Geometry: final body of the model. Coordinates: model frame, mm. Face numbers are marked on the shaded views. A direction names the side the tool comes from. Give positions to 0.01 mm unless a question says otherwise; leave off trailing zeros. Write each loop counter-clockwise with the first axis right and the second up, starting at its lowest first coordinate (ties: lowest second). Pieces come first, ordered by that corner, then holes.
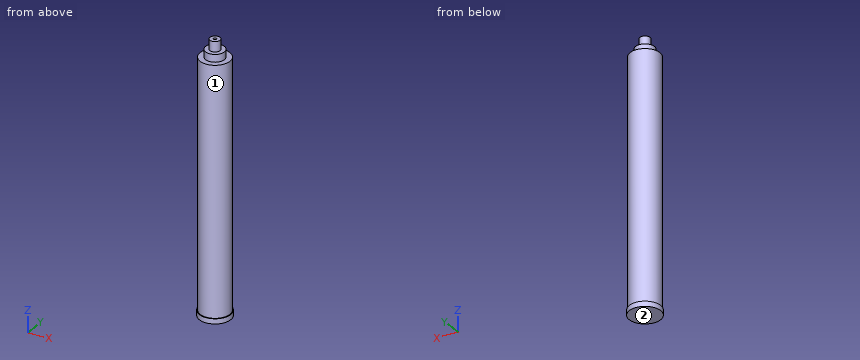
```python
from build123d import *

# Parameters (mm, degrees)
SKETCH1_R                   = 37.6555
BOSS_EXTRUDE1_DEPTH         = 621.03
SKETCH2_R                   = 39.6621
BOSS_EXTRUDE2_DEPTH         = 12.7
SKETCH4_R                   = 23.8125
BOSS_EXTRUDE4_DEPTH         = 19.05
SKETCH5_R                   = 12.7
BOSS_EXTRUDE5_DEPTH         = 25.4
F_3_8_16_TAPPED_HOLE1_D     = 7.9375
F_3_8_16_TAPPED_HOLE1_DEPTH = 25.4
F_3_8_16_TAPPED_HOLE1_TIP   = 2.384665582


with BuildPart() as part:
    # Sketch1 → Boss-Extrude1 (new body)
    with BuildSketch(Plane.XY):
        Circle(SKETCH1_R)
    extrude(amount=BOSS_EXTRUDE1_DEPTH)

    # Sketch2 → Boss-Extrude2 (add)
    with BuildSketch(Plane(origin=(0, 0, 0), x_dir=(-1, 0, 0), z_dir=(0, 0, -1))):
        Circle(SKETCH2_R)
    extrude(amount=BOSS_EXTRUDE2_DEPTH)

    # Sketch4 → Boss-Extrude4 (add)
    with BuildSketch(Plane.XY.offset(621.03)):
        Circle(SKETCH4_R)
    extrude(amount=BOSS_EXTRUDE4_DEPTH)

    # Sketch5 → Boss-Extrude5 (add)
    with BuildSketch(Plane.XY.offset(640.08)):
        Circle(SKETCH5_R)
    extrude(amount=BOSS_EXTRUDE5_DEPTH)

    # 3/8-16 Tapped Hole1
    with Locations(Plane.XY.offset(665.48)):
        with Locations((0, 0)):
            Hole(F_3_8_16_TAPPED_HOLE1_D / 2, depth=F_3_8_16_TAPPED_HOLE1_DEPTH)
            with Locations((0, 0, -(F_3_8_16_TAPPED_HOLE1_DEPTH + F_3_8_16_TAPPED_HOLE1_TIP / 2))):  # 118° drill point
                Cone(0, F_3_8_16_TAPPED_HOLE1_D / 2, F_3_8_16_TAPPED_HOLE1_TIP, mode=Mode.SUBTRACT)


solid = part.part
```
Item 1: Reachability of the marked faces 1 and 2 from +Z, -Z, +X, -X, +Y, -Y: full face, straight path, thin tool, end or side. Return the list, or none.
Found:
face 1: +Z
face 2: -Z, +X, -X, +Y, -Y
Item 2: Section A-A, the plane y = 32. Return the cut outline in (x, z), plus the area to 3 significant figures.
Found:
outline: (-23.43, -12.7) - (23.43, -12.7) - (23.43, 0) - (19.85, 0) - (19.85, 621.03) - (-19.85, 621.03) - (-19.85, 0) - (-23.43, 0) - close
area: 25,200 mm2
Item 3: Line query: L1, parallel to Y at x = 0, z = 655.5; L2, parallel to Y at x = 2.5, z = 566; L3, parallel to Y at x = -3, z = 384.5. Output: solid intervals per line, ascending.
Found:
L1: y = -12.7 to -3.97, 3.97 to 12.7
L2: y = -37.57 to 37.57
L3: y = -37.54 to 37.54
Item 4: Section B-B, the plane x = -30. Return the cut outline in (y, z).
Found:
outline: (-25.94, -12.7) - (25.94, -12.7) - (25.94, 0) - (22.76, 0) - (22.76, 621.03) - (-22.76, 621.03) - (-22.76, 0) - (-25.94, 0) - close
Item 5: Pin query (flat end, axial travel): pin 1 Ø24 at (x, y) = (12, 9) entering from +Z; pin 2 Ø3 at (y, z) = (-4, 190) entering from +X; pin 3 Ø8 at (y, z) = (12, 297) entering from -X; pin 4 Ø1 at (x, y) = (6.5, -29.5) entering from +Z. Return the tip coordinate at first contact, or that it passes through.
Found:
pin 1: stops at z = 665.48
pin 2: stops at x = 37.57
pin 3: stops at x = -36.8
pin 4: stops at z = 621.03
Item 6: Section C-C, the plane z = 112. Return the cut outline in (x, y).
Found:
outline: circle Ø75.31 at (0, 0)
